Could you check a few things on this model? Use its own coordinates, in mm. A direction names the side the tool comes from. Give positions to 0.01 mm unless a question says otherwise; leave off trailing zeros. Order: outer loops, then holes, each group sorted by start corner. A loop starts at its lowest first (then second) coordinate and runs counter-clockwise, first axis right, second up. Notation, with made-up numbers: (71.25, 28) -> (130.25, 28) arc R19 cw to (130.25, 43) -> close; hole circle Ø4 at (-28.5, 60.5). An arc over 180 degrees is marked (long way). One line per item, written item: value.
```python
from build123d import *

# Parameters (mm, degrees)
SKETCH1_W                  = 15
SKETCH1_H                  = 10
BOSS_EXTRUDE1_DEPTH        = 15
BOSS_EXTRUDE1_2_DEPTH      = 15
BOSS_EXTRUDE1_3_DEPTH      = 15
BOSS_EXTRUDE1_4_DEPTH      = 15
SKETCH2_W                  = 50
SKETCH2_H                  = 28
BOSS_EXTRUDE2_DEPTH        = 5
SKETCH4_W                  = 80
SKETCH4_H                  = 28
BOSS_EXTRUDE3_DEPTH        = 20
CUT_EXTRUDE1_DEPTH         = 20
CUT_EXTRUDE1_DEPTH_BACK    = 20
CUT_EXTRUDE2_DEPTH         = 1.25
M3_5_CLEARANCE_HOLE1_D     = 3.9
M3_5_CLEARANCE_HOLE1_DEPTH = 15
M3_5_CLEARANCE_HOLE1_TIP   = 1.171678207
FILLET1_R                  = 10
FILLET2_R                  = 5
FILLET3_R                  = 5


with BuildPart() as part:
    # Sketch1 → Boss-Extrude1 (new body)
    with BuildSketch(Plane(origin=(0, 0, 0), x_dir=(1, 0, 0), z_dir=(0, 1, 0))):
        with Locations((-17.5, 9)):
            Rectangle(SKETCH1_W, SKETCH1_H)
    extrude(amount=-BOSS_EXTRUDE1_DEPTH)



with BuildPart() as body_2:
    # Sketch1 → Boss-Extrude1 2 (new body)
    with BuildSketch(Plane(origin=(0, 0, 0), x_dir=(1, 0, 0), z_dir=(0, 1, 0))):
        with Locations((17.5, 9)):
            Rectangle(SKETCH1_W, SKETCH1_H)
    extrude(amount=-BOSS_EXTRUDE1_2_DEPTH)


with BuildPart() as body_3:
    # Sketch1 → Boss-Extrude1 3 (new body)
    with BuildSketch(Plane(origin=(0, 0, 0), x_dir=(1, 0, 0), z_dir=(0, 1, 0))):
        with Locations((17.5, -9)):
            Rectangle(SKETCH1_W, SKETCH1_H)
    extrude(amount=-BOSS_EXTRUDE1_3_DEPTH)


with BuildPart() as body_4:
    # Sketch1 → Boss-Extrude1 4 (new body)
    with BuildSketch(Plane(origin=(0, 0, 0), x_dir=(1, 0, 0), z_dir=(0, 1, 0))):
        with Locations((-17.5, -9)):
            Rectangle(SKETCH1_W, SKETCH1_H)
    extrude(amount=-BOSS_EXTRUDE1_4_DEPTH)


with BuildPart() as part_1:
    add(part.part)

    add(body_2.part)  # Boss-Extrude2 merges body 2

    add(body_3.part)  # Boss-Extrude2 merges body 3

    add(body_4.part)  # Boss-Extrude2 merges body 4
    # Sketch2 → Boss-Extrude2 (add)
    with BuildSketch(Plane(origin=(0, 0, 0), x_dir=(1, 0, 0), z_dir=(0, 1, 0))):
        Rectangle(SKETCH2_W, SKETCH2_H)
    extrude(amount=BOSS_EXTRUDE2_DEPTH)

    # Sketch4 → Boss-Extrude3 (add)
    with BuildSketch(Plane(origin=(0, 0, 0), x_dir=(1, 0, 0), z_dir=(0, 1, 0))):
        Rectangle(SKETCH4_W, SKETCH4_H)
    extrude(amount=BOSS_EXTRUDE3_DEPTH)

    # Sketch5 → Cut-Extrude1 (cut, two sides: drawn at the far end of the back side and taken through both)
    with BuildSketch(Plane.XY.offset(-CUT_EXTRUDE1_DEPTH_BACK)):
        Polygon((-25, 20), (25, 20), (0, 5), align=None)
    extrude(amount=CUT_EXTRUDE1_DEPTH + CUT_EXTRUDE1_DEPTH_BACK, mode=Mode.SUBTRACT)

    # Sketch6 → Cut-Extrude2 (cut, symmetric)
    with BuildSketch(Plane.XY):
        Polygon((-25, 20), (-25, 5), (0, 5), align=None)
    cut_extrude2 = extrude(amount=CUT_EXTRUDE2_DEPTH, both=True, mode=Mode.SUBTRACT)

    # Mirror1: Cut-Extrude2 across plane
    add(cut_extrude2.mirror(Plane(origin=(0, 0, 0), x_dir=(0, 0, 1), z_dir=(1, 0, 0))), mode=Mode.SUBTRACT)

    # M3.5 Clearance Hole1
    with Locations(Plane(origin=(0, 20, 0), x_dir=(1, 0, 0), z_dir=(0, 1, 0))):
        with Locations((32.5, 0), (-32.5, 0)):
            Hole(M3_5_CLEARANCE_HOLE1_D / 2, depth=M3_5_CLEARANCE_HOLE1_DEPTH)
            with Locations((0, 0, -(M3_5_CLEARANCE_HOLE1_DEPTH + M3_5_CLEARANCE_HOLE1_TIP / 2))):  # 118° drill point
                Cone(0, M3_5_CLEARANCE_HOLE1_D / 2, M3_5_CLEARANCE_HOLE1_TIP, mode=Mode.SUBTRACT)

    # Fillet1
    fillet1_edges = [part_1.edges().sort_by_distance(p)[0] for p in [
        (-25, 0, -9),
        (-25, 0, 9),
        (25, 0, 9),
        (25, 0, -9),
    ]]
    fillet(fillet1_edges, radius=FILLET1_R)

    # Fillet2
    fillet2_edges = [part_1.edges().sort_by_distance(p)[0] for p in [
        (10, 0, -9),
        (10, 0, 9),
        (-10, 0, 9),
        (-10, 0, -9),
    ]]
    fillet(fillet2_edges, radius=FILLET2_R)

    # Fillet3
    fillet3_edges = [part_1.edges().sort_by_distance(p)[0] for p in [
        (-40, 10, -14),
        (-40, 10, 14),
        (40, 10, 14),
        (40, 10, -14),
    ]]
    fillet(fillet3_edges, radius=FILLET3_R)


solid = part_1.part
```
1) Suppose I cut it at D-D, the plane z = 7.25. Write out the boundary of the cut face in (x, y), then the cut area to 3 significant figures.
Answer below:
outline: (-40, 0) -> (-35, 0) arc R10 cw to (-25, -10) -> (-25, -15) -> (-10, -15) -> (-10, -5) arc R5 cw to (-5, 0) -> (5, 0) arc R5 cw to (10, -5) -> (10, -15) -> (25, -15) -> (25, -10) arc R10 cw to (35, 0) -> (40, 0) -> (40, 20) -> (25, 20) -> (0, 5) -> (-25, 20) -> (-40, 20) -> close
area: 1,730 mm2
2) If I drill on line 1 along Z through (x, y) = (-32.5, 16.25); line 2 along Z through (x, y) = (-6, 8.5); line 3 along Y through (x, z) = (-36, 3.5), over which ranges is the centre line in solid material (lowest first)?
Answer below:
line 1: z = -14 to -1.95, 1.95 to 14
line 2: z = -14 to -1.25, 1.25 to 14
line 3: y = 0 to 20
3) Suppose I cut it at B-B, the plane x = -9. Write out the boundary of the cut face in (y, z), then the cut area to 3 significant figures.
Answer below:
outline: (-2, -14) -> (10.4, -14) -> (10.4, -1.25) -> (5, -1.25) -> (5, 1.25) -> (10.4, 1.25) -> (10.4, 14) -> (-2, 14) -> (-2, 4) -> (0, 4) -> (0, -4) -> (-2, -4) -> close
area: 318 mm2
4) We'd pull the mould along Z, two halves only. Please class faces 4 (the cylindrical face through (-38, 10, 13)), 5 (the flat face through (18, 9, 1.25)), 6 (the flat face through (12.675, 12.605, -7.714)): +Z half, -Z half, draft (parallel to the pull), parting line (faces both ways), or undercut.
Answer below:
face 4: +Z half
face 5: undercut
face 6: draft
5) For faces 1 (the flat face through (-25, -13, 9)), 2 (the cylindrical face through (-9, -2, 9)), 3 (the flat face through (25, -13, -9)), which set-ups out of +Z, -Z, +X, -X, +Y, -Y let a thin tool reach every point of the face, with its end or its side?
Answer below:
face 1: +Z, -Z, -X, -Y
face 2: +Z, -Z, -Y
face 3: +Z, -Z, +X, -Y
6) For P1, Ø8, axis at y = -10, z = -11, coming from the -X side; P2, Ø3, axis at y = -8, z = 8, coming from the -X side; P3, Ø3, axis at y = -10, z = -8.5, coming from the +X side, each with a flat end and sliding along its axis, tell me the tip position at first contact or that it passes through.
Answer below:
P1: stops at x = -25.83
P2: stops at x = -25.63
P3: stops at x = 25.11
7) Suppose I cut it at A-A, the plane y = 9. Write out the boundary of the cut face in (x, z).
Answer below:
outline: (-40, -9) arc R5 ccw to (-35, -14) -> (-6.67, -14) -> (-6.67, -1.25) -> (-25, -1.25) -> (-25, 1.25) -> (-6.67, 1.25) -> (-6.67, 14) -> (-35, 14) arc R5 ccw to (-40, 9) -> close; (6.67, -14) -> (35, -14) arc R5 ccw to (40, -9) -> (40, 9) arc R5 ccw to (35, 14) -> (6.67, 14) -> (6.67, 1.25) -> (25, 1.25) -> (25, -1.25) -> (6.67, -1.25) -> close; hole circle Ø3.9 at (-32.5, 0); hole circle Ø3.9 at (32.5, 0)
8) Suppose I cut it at C-C, the plane z = 3. Write out the boundary of the cut face in (x, y), then the cut area to 4 significant figures.
Answer below:
outline: (-40, 0) -> (40, 0) -> (40, 20) -> (25, 20) -> (0, 5) -> (-25, 20) -> (-40, 20) -> close
area: 1,225 mm2
